```python
from build123d import *

# Parameters (mm, degrees)
CROQUIS1_W                                   = 260
CROQUIS1_H                                   = 80
BRIDA_BASE1_DEPTH                            = 6.35
REDONDEO1_R                                  = 2
TALADRO_DE_MARGEN_PARA_M51_D                 = 5.5
REFRENTADO_PARA_TORNILLO_TAP_N_CON_C_2_COUNT = 2
REFRENTADO_PARA_TORNILLO_TAP_N_CON_C_2_PITCH = 44
REFRENTADO_PARA_TORNILLO_TAP_N_CON_C_3_COUNT = 2
REFRENTADO_PARA_TORNILLO_TAP_N_CON_C_3_PITCH = 60.827625303
REFRENTADO_PARA_TORNILLO_TAP_N_CON_C_4_COUNT = 2
REFRENTADO_PARA_TORNILLO_TAP_N_CON_C_4_PITCH = 42
CROQUIS11_R                                  = 20
CORTAR_EXTRUIR1_DEPTH                        = 10


# Sheet-metal steps are written as plain solids
with BuildPart() as part:
    # Croquis1 → Brida base1 (new body)
    with BuildSketch(Plane(origin=(0, 0, 0), x_dir=(1, 0, 0), z_dir=(0, 1, 0))):
        with Locations((-19.777777778, -5.555555556)):
            Rectangle(CROQUIS1_W, CROQUIS1_H)
    extrude(amount=-BRIDA_BASE1_DEPTH)

    # Redondeo1
    redondeo1_edges = [part.edges().sort_by_distance(p)[0] for p in [
        (-149.777777778, -3.175, -34.444444444),
        (110.222222222, -3.175, -34.444444444),
        (110.222222222, -3.175, 45.555555556),
        (-149.777777778, -3.175, 45.555555556),
    ]]
    fillet(redondeo1_edges, radius=REDONDEO1_R)

    # Taladro de margen para M51 (through all)
    with Locations(Plane(origin=(0, 0, 0), x_dir=(1, 0, 0), z_dir=(0, 1, 0))):
        with Locations((-119.777777778, 24.444444444), (-119.777777778, -35.555555556), (80.222222222, -35.555555556), (80.222222222, 24.444444444)):
            Hole(TALADRO_DE_MARGEN_PARA_M51_D / 2)

    # Croquis9 → Refrentado para tornillo tapón con cabeza plana de clavija de M61 (revolve, cut)
    with BuildSketch(Plane(origin=(-41.777777778, 0, -15.444444444), x_dir=(0, 0, 1), z_dir=(1, 0, 0))):
        Polygon((0, 0), (0, 6.35), (3.3, 6.35), (3.3, 3.42), (6.72, 0), align=None)
    refrentado_para_tornillo_tap_n_con_cabez = revolve(axis=Axis((-41.777777778, 6.35, -15.444444444), (0, -1, 0)), mode=Mode.SUBTRACT)

    # Refrentado para tornillo tap_n con c 2: Refrentado para tornillo tapón con cabeza plana de clavija de M61 ×2
    with Locations(*[(i * REFRENTADO_PARA_TORNILLO_TAP_N_CON_C_2_PITCH, 0, 0) for i in range(1, REFRENTADO_PARA_TORNILLO_TAP_N_CON_C_2_COUNT)]):
        add(refrentado_para_tornillo_tap_n_con_cabez, mode=Mode.SUBTRACT)

    # Refrentado para tornillo tap_n con c 3: Refrentado para tornillo tapón con cabeza plana de clavija de M61 ×2
    with Locations(*[Vector(0.7233555441435721, 0, 0.6904757466825007) * (i * REFRENTADO_PARA_TORNILLO_TAP_N_CON_C_3_PITCH) for i in range(1, REFRENTADO_PARA_TORNILLO_TAP_N_CON_C_3_COUNT)]):
        add(refrentado_para_tornillo_tap_n_con_cabez, mode=Mode.SUBTRACT)

    # Refrentado para tornillo tap_n con c 4: Refrentado para tornillo tapón con cabeza plana de clavija de M61 ×2
    with Locations(*[(0, 0, i * REFRENTADO_PARA_TORNILLO_TAP_N_CON_C_4_PITCH) for i in range(1, REFRENTADO_PARA_TORNILLO_TAP_N_CON_C_4_COUNT)]):
        add(refrentado_para_tornillo_tap_n_con_cabez, mode=Mode.SUBTRACT)

    # Croquis11 → Cortar-Extruir1 (cut)
    with BuildSketch(Plane(origin=(0, 0, 0), x_dir=(1, 0, 0), z_dir=(0, 1, 0))):
        with Locations(Location((-89.777777778, -5.555555556, 0), (0, 0, 270))):
            Circle(CROQUIS11_R)
        with Locations(Location((50.222222222, -5.555555556, 0), (0, 0, 270))):
            Circle(CROQUIS11_R)
    extrude(amount=-CORTAR_EXTRUIR1_DEPTH, mode=Mode.SUBTRACT)


solid = part.part
```
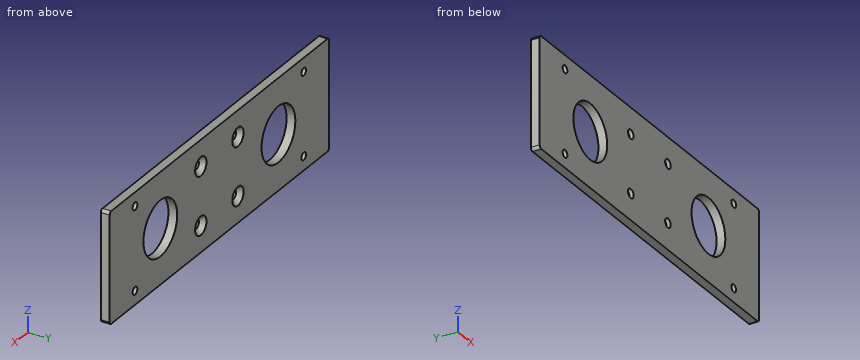
Check sheet for the modelled part. Datum: model origin and axes. Units: mm. Coordinates: 2 decimals unless noted, no trailing zeros. Write each loop counter-clockwise with the first axis right and the second up, starting at its lowest first coordinate (ties: lowest second). Pieces come first, ordered by that corner, then holes. Notation, with made-up numbers: (56.25, 6.5) - (77.25, 6.5) arc R20 cw to (77.25, 37.5) - close; hole circle Ø6 at (-5.75, 73). An arc over 180 degrees is marked (long way). One line per question, with ' | ' between items.
Item 1: Sectioned sample at A-A on z = 14. Record the boundary of the cut face in (x, y).
Determined:
outline: (-149.78, -6.35) - (-107.91, -6.35) - (-107.91, 0) - (-149.78, 0) - close; (-71.65, -6.35) - (32.09, -6.35) - (32.09, 0) - (-71.65, 0) - close; (68.35, -6.35) - (110.22, -6.35) - (110.22, 0) - (68.35, 0) - close
Item 2: Thickness scan on line 1 (X direction, y = -4.5, z = -15.5); line 2 (X direction, y = -5, z = 33.5); line 3 (Z direction, x = -118, y = -5.25). Record the ranges inside material, lowest first. Write a range as [from, to].
Determined:
line 1: x = [-149.78, -45.08], [-38.48, -1.08], [5.52, 110.22] | line 2: x = [-149.78, -121.6], [-117.95, 78.4], [82.05, 110.22] | line 3: z = [-34.44, -26.54], [-22.35, 33.46], [37.65, 45.56]
Item 3: Sectioned sample at C-C on y = -2. Give the number of separate pieces and of enclosed holes in the cut face, plus the area to 3 significant figures.
Determined:
separate pieces: 1 | enclosed holes: 10 | area: 17,900 mm2
Item 4: Sectioned sample at B-B on x = -83. Record the boundary of the cut face in (y, z), plus the area to 3 significant figures.
Determined:
outline: (-6.35, -34.44) - (0, -34.44) - (0, -13.26) - (-6.35, -13.26) - close; (-6.35, 24.37) - (0, 24.37) - (0, 45.56) - (-6.35, 45.56) - close | area: 269 mm2
Item 5: Gauge pin test, flat end, axial feed: P1, Ø8.5, axis at x = -41.78, z = 26.56, coming from the +Y side. Record the tip position at first contact, or that the pin passes through.
Determined:
P1: stops at y = -2.47
Item 6: Sectioned sample at D-D on z = -5.5. Record the boundary of the cut face in (x, y), plus the area to 3 significant figures.
Determined:
outline: (-149.78, -6.35) - (-106.44, -6.35) - (-106.44, 0) - (-149.78, 0) - close; (-73.11, -6.35) - (33.56, -6.35) - (33.56, 0) - (-73.11, 0) - close; (66.89, -6.35) - (110.22, -6.35) - (110.22, 0) - (66.89, 0) - close | area: 1,230 mm2
